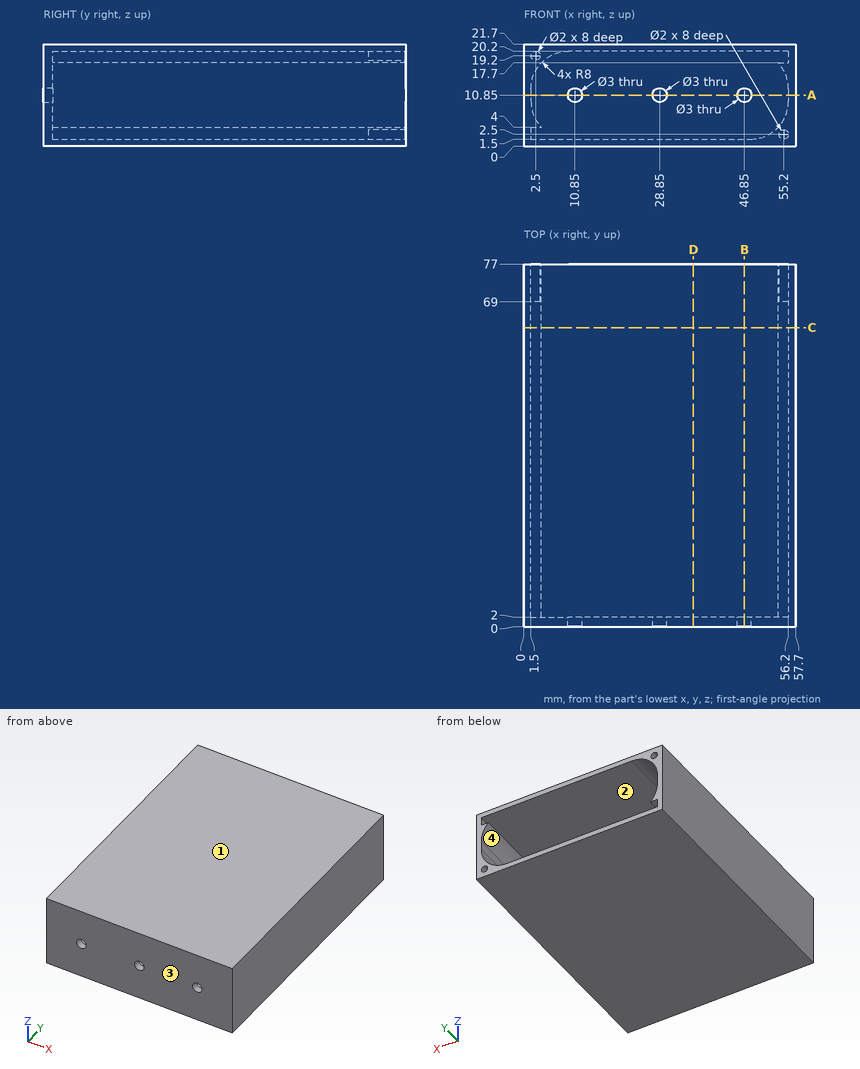
Geometry: see drawing. Coordinates: mm, zero at the bounding-box minimum. Coordinates: 2 decimals unless noted, no trailing zeros. Order: outer loops, then holes, each group sorted by start corner. A loop starts at its lowest first (then second) coordinate and runs counter-clockwise, first axis right, second up. Notation, with made-up numbers: (47.25, 79.25) -> (85.25, 79.25) arc R20 ccw to (85.25, 97.25) -> close; hole circle Ø7 at (59, -1). An arc over 180 degrees is marked (long way). Write each question's results on one line, items separated by ' | '. Start each with the question number.
1) Cut plane D-D, the plane x = 36. Output: boundary loops of the cut face in (y, z), and give its area (3 significant figures).
2) Cut plane A-A, the plane z = 10.85. Output: boundary loops of the cut face in (x, y), and give its area (3 significant figures).
3) Material intervals for line 1 along X through (y, z) = (26.5, 17.5); line 2 along X through (y, z) = (0.85, 10.85); line 3 along Z through (x, y) = (24, 65), sorted ascending.
4) First-contact query: pin 1 (0.7 mm diameter, centred on x = 3, y = 30, fed in from -Z); pin 2 (8 mm diameter, centred on x = 19, z = 6, fed in from +Y). Flat tips, straight axial feed; report the tip coordinate or a pass-through.
5) Cut plane B-B, the plane x = 46.85. Output: boundary loops of the cut face in (y, z), and give its area (3 significant figures).
6) Mould query, pull axis Z, two halves, no side actions, for the marked faces 1, 2, 3 and 4. Classes: released by +Z, released by -Z, zero draft, split by the parting line, or undercut.
7) Cut plane C-C, the plane y = 63.5. Output: boundary loops of the cut face in (x, z), and give its area (3 significant figures).
Checks:
1) outline: (0, 0) -> (77, 0) -> (77, 1.5) -> (2, 1.5) -> (2, 20.2) -> (77, 20.2) -> (77, 21.7) -> (0, 21.7) -> close | area: 268 mm^2
2) outline: (0, 0) -> (9.35, 0) -> (9.35, 2) -> (1.5, 2) -> (1.5, 77) -> (0, 77) -> close; (12.35, 0) -> (27.35, 0) -> (27.35, 2) -> (12.35, 2) -> close; (30.35, 0) -> (45.35, 0) -> (45.35, 2) -> (30.35, 2) -> close; (48.35, 0) -> (57.7, 0) -> (57.7, 77) -> (56.2, 77) -> (56.2, 2) -> (48.35, 2) -> close | area: 322 mm^2
3) line 1: 0 to 3.51, 54.19 to 57.7 | line 2: 0 to 9.35, 12.35 to 27.35, 30.35 to 45.35, 48.35 to 57.7 | line 3: 0 to 1.5, 20.2 to 21.7
4) pin 1: z = 0 | pin 2: y = 2
5) outline: (0, 0) -> (77, 0) -> (77, 1.5) -> (2, 1.5) -> (2, 9.35) -> (0, 9.35) -> close; (0, 12.35) -> (2, 12.35) -> (2, 20.2) -> (77, 20.2) -> (77, 21.7) -> (0, 21.7) -> close | area: 262 mm^2
6) face 1: released by +Z | face 2: undercut | face 3: zero draft | face 4: undercut
7) outline: (0, 0) -> (57.7, 0) -> (57.7, 21.7) -> (0, 21.7) -> close; hole (1.5, 1.5) -> (48.2, 1.5) arc R8 ccw to (56.2, 9.5) -> (56.2, 12.2) arc R8 ccw to (54.01, 17.7) -> (56.2, 17.7) -> (56.2, 20.2) -> (9.5, 20.2) arc R8 ccw to (1.5, 12.2) -> (1.5, 9.5) arc R8 ccw to (3.69, 4) -> (1.5, 4) -> close | area: 264 mm^2
